Check sheet for the modelled part. Datum: model origin and axes. Units: mm. Face numbers are marked on the shaded views. A direction names the side the tool comes from. Round coordinates to 2 decimals unless told otherwise and drop trailing zeros. Write each loop counter-clockwise with the first axis right and the second up, starting at its lowest first coordinate (ties: lowest second). Pieces come first, ordered by that corner, then holes. Notation, with made-up numbers: (-10, -28.5) -> (36, -28.5) arc R20 cw to (36, -4.5) -> close; hole circle Ø3 at (66, 2). An arc over 180 degrees is marked (long way). Answer as a JSON object with one key per item and string values. Group by question number.
```python
from build123d import *

# Parameters (mm, degrees)
F1_W     = 114.3
F1_H     = 66.04
F2_DEPTH = 8.89
F3_W     = 127
F3_H     = 78.74
F3_W_2   = 114.3
F3_H_2   = 66.04
F4_DEPTH = 19.05
F5_W     = 127
F5_H     = 78.74
F6_DEPTH = 6.35


with BuildPart() as f2:
    # F1 (on Top) → F2 (new body)
    with BuildSketch(Plane.XY):
        Polygon((-63.5, 0), (-63.5, -55.88), (-63.5, -134.62), (63.5, -134.62), (63.5, -55.88), (63.5, 0), (26.67, 0), (26.67, -55.88), (-26.67, -55.88), (-26.67, 0), align=None)
        with Locations((0, -95.25)):
            Rectangle(F1_W, F1_H, mode=Mode.SUBTRACT)
    extrude(amount=F2_DEPTH)

    # F3 (on Top) → F4 (join)
    with BuildSketch(Plane.XY):
        with Locations((0, -95.25)):
            Rectangle(F3_W, F3_H)
        with Locations((0, -95.25)):
            Rectangle(F3_W_2, F3_H_2, mode=Mode.SUBTRACT)
    extrude(amount=-F4_DEPTH)

    # F5 (on face) → F6 (join)
    with BuildSketch(Plane(origin=(0, 0, -19.05), x_dir=(1, 0, 0), z_dir=(0, 0, -1))):
        with Locations((0, 95.25)):
            Rectangle(F5_W, F5_H)
    extrude(amount=F6_DEPTH)

    # F7: F2 across plane


with BuildPart() as f2_1:
    add(f2.part)
    add(f2.part.mirror(Plane.XZ))


solid = f2_1.part
```
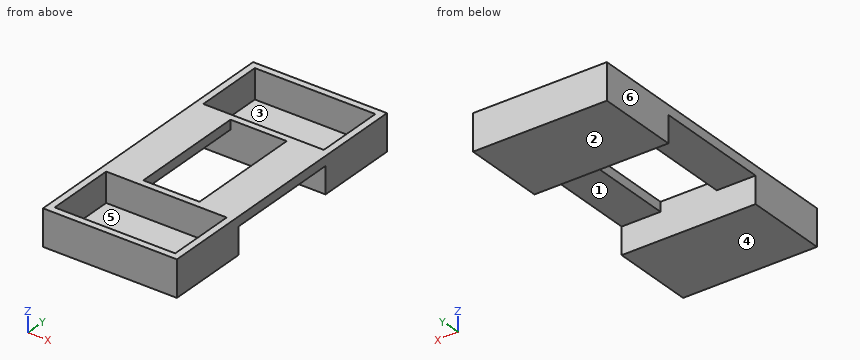
(1) Section check A-A on y = -37. Record the cut outline in (x, z).
(2) Section check B-B on z = -15.5. Record the cut outline in (x, y), then the cut area to 3 significant figures.
(3) Section check D-D on y = -109. Record the cut outline in (x, z), then the cut area to 3 significant figures.
(4) Release check for a two-part mould opening along X. For the marked faces 4, 5 and 6 record: pulls with the +X half, pulls with the -X half, needs draft (parallel to the pull), parting line crosses it, or undercut.
(5) Access from +Z, -Z, +X, -X, +Y, -Y to the whole of each face (thin tool, end or side, straight path). Record for the marked faces 1, 2 and 3.
(6) Scan lines: line 1 along Y through (x, z) = (48.5, -0.5); line 2 along X through (y, z) = (84, -3.5); line 3 along X through (y, z) = (5.5, 1). Record each from-to range of solid material in increasing order.
(7) Section check C-C on x = 16. Record the cut outline in (y, z), then the cut area to 3 significant figures.
(8) Go/stop test with flat-tipped pins: pin 1 Ø20 at (x, y) = (12, 89.5) entering from +Z; pin 2 Ø11 at (x, y) = (-54, 0) entering from -Z. Record where each tip stops, or that it passes through.
Data:
{
 "1": {"outline": "(-63.5, 0) -> (-26.67, 0) -> (-26.67, 8.89) -> (-63.5, 8.89) -> close; (26.67, 0) -> (63.5, 0) -> (63.5, 8.89) -> (26.67, 8.89) -> close"},
 "2": {"outline": "(-63.5, -134.62) -> (63.5, -134.62) -> (63.5, -55.88) -> (-63.5, -55.88) -> close; (-63.5, 55.88) -> (63.5, 55.88) -> (63.5, 134.62) -> (-63.5, 134.62) -> close; hole (-57.15, -128.27) -> (57.15, -128.27) -> (57.15, -62.23) -> (-57.15, -62.23) -> close; hole (-57.15, 62.23) -> (57.15, 62.23) -> (57.15, 128.27) -> (-57.15, 128.27) -> close", "area": "4,900 mm²"},
 "3": {"outline": "(-63.5, -25.4) -> (63.5, -25.4) -> (63.5, 8.89) -> (57.15, 8.89) -> (57.15, -19.05) -> (-57.15, -19.05) -> (-57.15, 8.89) -> (-63.5, 8.89) -> close", "area": "1,160 mm²"},
 "4": {"face 4": "needs draft", "face 5": "undercut", "face 6": "pulls with the -X half"},
 "5": {"face 1": "-Z, +X, -X", "face 2": "-Z, +X, -X, +Y, -Y", "face 3": "+Z"},
 "6": {"line 1": "y = -134.62 to -128.27, -62.23 to -55.88, 55.88 to 62.23, 128.27 to 134.62", "line 2": "x = -63.5 to -57.15, 57.15 to 63.5", "line 3": "x = -63.5 to -26.67, 26.67 to 63.5"},
 "7": {"outline": "(-134.62, -25.4) -> (-55.88, -25.4) -> (-55.88, 8.89) -> (-62.23, 8.89) -> (-62.23, -19.05) -> (-128.27, -19.05) -> (-128.27, 8.89) -> (-134.62, 8.89) -> close; (55.88, -25.4) -> (134.62, -25.4) -> (134.62, 8.89) -> (128.27, 8.89) -> (128.27, -19.05) -> (62.23, -19.05) -> (62.23, 8.89) -> (55.88, 8.89) -> close", "area": "1,710 mm²"},
 "8": {"pin 1": "stops at z = -19.05", "pin 2": "stops at z = 0"}
}
